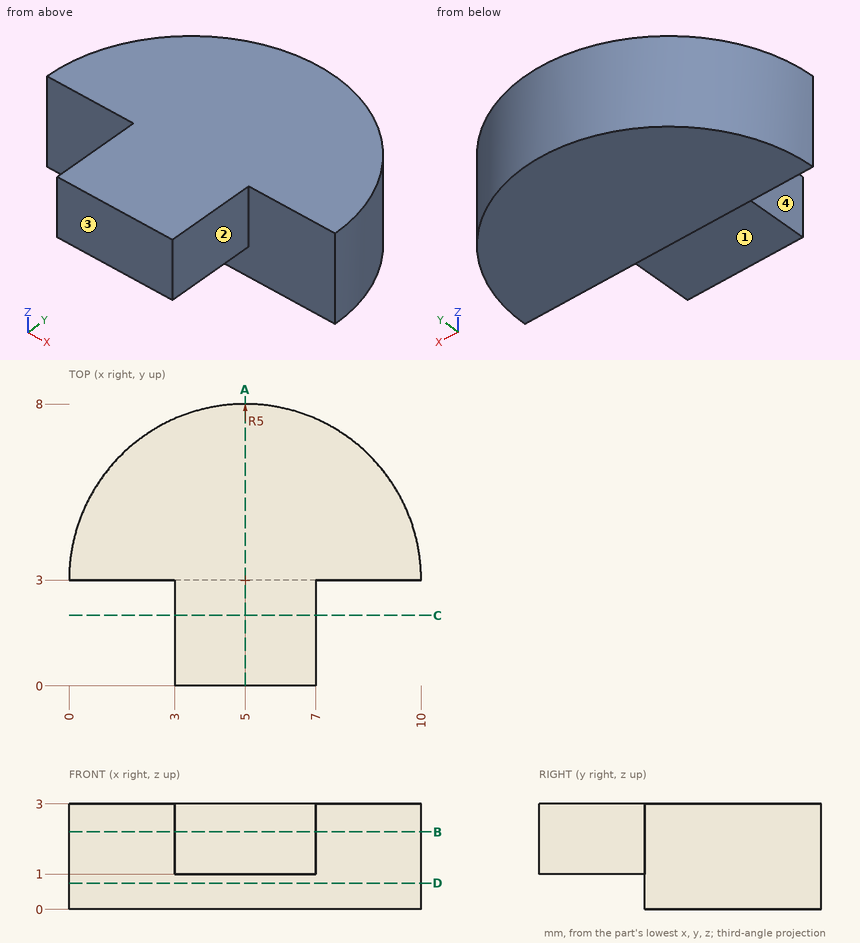
Could you check a few things on this drawing? It's one solid part, dimensions in mm from its lowest x, y, z. A direction names the side the tool comes from. Give positions to 0.01 mm unless a question says otherwise; leave off trailing zeros. Loops run counter-clockwise (first coordinate to the right, second up) from the corner with the lowest first, then second, coordinate; pieces in that order, holes last. Notation, with made-up numbers: (-10, 35) -> (18, 35) arc R10 cw to (18, 41) -> close; hole circle Ø1 at (67.25, -23.75). An arc over 180 degrees is marked (long way). Answer as CSV lines item,"result". Start each with the question number.
(1) I need wall thicknesses on probe 1 along X at (y, z) = (2.75, 2); probe 2 along Z at (x, y) = (4.25, 1.75); probe 3 along Y at (x, z) = (4.75, 0.25). Which ranges of each line are inside material? Lowest first, please.
(2) If we section it at D-D on z = 0.75: Write out the boundary of the cut face in (x, y).
(3) Which directions (+Z, -Z, +X, -X, +Y, -Y) give clear straight access to the entire face, cutting with the end or side of a thin tool? Please do the marked faces 1, 2, 3 and 4.
(4) I'm going to push flat-ended pins straight in: pin 1 Ø1 at (y, z) = (4, 0.5) entering from -X; pin 2 Ø0.9 at (x, y) = (4, 1.5) entering from -Z; pin 3 Ø0.6 at (y, z) = (1, 1.5) entering from -X. Where does each tip first touch, or does it pass through?
(5) If we section it at A-A on x = 5: Write out the boundary of the cut face in (y, z), then the cut area to 3 significant figures.
(6) If we section it at C-C on y = 2: Write out the boundary of the cut face in (x, z), then the cut area to 3 significant figures.
(7) If we section it at B-B on z = 2.2: Write out the boundary of the cut face in (x, y), then the cut area to 3 significant figures.
Computed:
1,probe 1,"x = 3 to 7"
1,probe 2,"z = 1 to 3"
1,probe 3,"y = 3 to 7.99"
2,outline,"(0, 3) -> (10, 3) arc R5 ccw to start"
3,face 1,"-Z, +X, -X, -Y"
3,face 2,"+Z, -Z, +X, -Y"
3,face 3,"+Z, -Z, +X, -X, -Y"
3,face 4,"+Z, -Z, -X, -Y"
4,pin 1,"stops at x = 0.03"
4,pin 2,"stops at z = 1"
4,pin 3,"stops at x = 3"
5,outline,"(0, 1) -> (3, 1) -> (3, 0) -> (8, 0) -> (8, 3) -> (0, 3) -> close"
5,area,"21.0 mm2"
6,outline,"(3, 1) -> (7, 1) -> (7, 3) -> (3, 3) -> close"
6,area,"8.00 mm2"
7,outline,"(0, 3) -> (3, 3) -> (3, 0) -> (7, 0) -> (7, 3) -> (10, 3) arc R5 ccw to start"
7,area,"51.3 mm2"
